```python
from build123d import *

# Parameters (mm, degrees)
SKETCH_1_R               = 12.5
EXTRUDE_1_DEPTH          = 6
SKETCH_4_R               = 1.15
CUT_EXTRUDE_2_DEPTH      = 19
SKETCH_3_R               = 7.5
CUT_EXTRUDE_3_DEPTH      = 5
CHAMFER_2_SIZE           = 0.7
SKETCH_8_R               = 17.454292773
SKETCH_8_R_2             = 8.65
CUT_EXTRUDE_4_DEPTH      = 3
PATTERN_CIRCULAR_2_COUNT = 6
SKETCH_2_R               = 7.34982993
EXTRUDE_2_DEPTH          = 10
SKETCH_9_R               = 1.85
CUT_EXTRUDE_5_DEPTH      = 0.3
CHAMFER_3_SIZE           = 0.7
PATTERN_CIRCULAR_3_COUNT = 6
CHAMFER_4_SIZE           = 0.7
SKETCH_10_W              = 4.08
SKETCH_10_H              = 4.08
CUT_EXTRUDE_6_DEPTH      = 8
FILLET_1_R               = 2
CHAMFER_5_SIZE           = 4.08


# Some blends are built 0.0001 mm under size
with BuildPart() as part:
    # 草图1 → 凸台-拉伸1 (new body)
    with BuildSketch(Plane(origin=(0, 0, 0), x_dir=(1, 0, 0), z_dir=(0, 1, 0))):
        with Locations(Location((0, 0, 0), (0, 0, 270))):
            Circle(SKETCH_1_R)
    extrude(amount=EXTRUDE_1_DEPTH)

    # 草图4 → 切除-拉伸2 (cut)
    with BuildSketch(Plane(origin=(0, 6, 0), x_dir=(1, 0, 0), z_dir=(0, 1, 0))):
        with Locations(Location((-10.5, 0, 0), (0, 0, 270))):
            Circle(SKETCH_4_R)
    cut_extrude_2 = extrude(amount=-CUT_EXTRUDE_2_DEPTH, mode=Mode.SUBTRACT)

    # 草图3 → 切除-拉伸3 (cut)
    with BuildSketch(Plane(origin=(0, 0, 0), x_dir=(-1, 0, 0), z_dir=(0, -1, 0))):
        with Locations(Location((0, 0, 0), (0, 0, 90))):
            Circle(SKETCH_3_R)
    extrude(amount=-CUT_EXTRUDE_3_DEPTH, mode=Mode.SUBTRACT)

    # 倒角2
    chamfer_2_edges = [part.edges().sort_by_distance(p)[0] for p in [
        (-10.5, 6, -1.15),
    ]]
    chamfer(chamfer_2_edges, length=CHAMFER_2_SIZE)

    # 草图8 → 切除-拉伸4 (cut)
    with BuildSketch(Plane(origin=(0, 6, 0), x_dir=(1, 0, 0), z_dir=(0, 1, 0))):
        Circle(SKETCH_8_R)
        with Locations(Location((0, 0, 0), (0, 0, 270))):
            Circle(SKETCH_8_R_2, mode=Mode.SUBTRACT)
    extrude(amount=-CUT_EXTRUDE_4_DEPTH, mode=Mode.SUBTRACT)

    # 阵列(圆周)2: 切除-拉伸2 ×6 about axis
    pattern_circular_2_axis = Axis((0, 0, 0), (0, 1, 0))
    for i in range(1, PATTERN_CIRCULAR_2_COUNT):
        add(cut_extrude_2.rotate(pattern_circular_2_axis, i * 360 / PATTERN_CIRCULAR_2_COUNT), mode=Mode.SUBTRACT)

    # 草图2 → 凸台-拉伸2 (add)
    with BuildSketch(Plane(origin=(0, 6, 0), x_dir=(1, 0, 0), z_dir=(0, 1, 0))):
        with Locations(Location((0, 0, 0), (0, 0, 270))):
            Circle(SKETCH_2_R)
    extrude(amount=EXTRUDE_2_DEPTH)

    # 草图9 → 切除-拉伸5 (cut)
    with BuildSketch(Plane(origin=(0, 3, 0), x_dir=(1, 0, 0), z_dir=(0, 1, 0))):
        with Locations(Location((-10.5, 0, 0), (0, 0, 270))):
            Circle(SKETCH_9_R)
    cut_extrude_5 = extrude(amount=-CUT_EXTRUDE_5_DEPTH, mode=Mode.SUBTRACT)

    # 倒角3
    chamfer_3_edges = [part.edges().sort_by_distance(p)[0] for p in [
        (-10.5, 2.7, -1.15),
    ]]
    chamfer(chamfer_3_edges, length=CHAMFER_3_SIZE - 0.0001)  # a hair under: the kernel refuses the full size

    # 阵列(圆周)3: 切除-拉伸5 ×6 about axis
    pattern_circular_3_axis = Axis((0, 0, 0), (0, 1, 0))
    for i in range(1, PATTERN_CIRCULAR_3_COUNT):
        add(cut_extrude_5.rotate(pattern_circular_3_axis, i * 360 / PATTERN_CIRCULAR_3_COUNT), mode=Mode.SUBTRACT)

    # 倒角4
    chamfer_4_edges = [part.edges().sort_by_distance(p)[0] for p in [
        (-4.254070786, 2.7, -9.66826674),
        (6.245929214, 2.7, -8.51826674),
        (10.5, 2.7, 1.15),
        (4.254070786, 2.7, 9.66826674),
        (-6.245929214, 2.7, 8.51826674),
    ]]
    chamfer(chamfer_4_edges, length=CHAMFER_4_SIZE - 0.0001)  # a hair under: the kernel refuses the full size

    # 草图10 → 切除-拉伸6 (cut)
    with BuildSketch(Plane(origin=(0, 16, 0), x_dir=(1, 0, 0), z_dir=(0, 1, 0))):
        Rectangle(SKETCH_10_W, SKETCH_10_H)
    extrude(amount=-CUT_EXTRUDE_6_DEPTH, mode=Mode.SUBTRACT)

    # 草图11 → 切除-旋转1 (revolve, cut)
    with BuildSketch(Plane(origin=(0, 0, 0), x_dir=(0, 0, -1), z_dir=(1, 0, 0)), mode=Mode.PRIVATE) as cut_revolve_1_sk:
        Polygon((-0.304897272, 10.075), (-10.874100718, 10.075), (-10.874100718, 6), (-3.64, 6), (-3.64, 7.875), (-2.04, 7.875), (-2.04, 9.125), (11.125701635, 9.125), (11.125701635, 10.075), align=None)
    revolve(cut_revolve_1_sk.sketch.rotate(Axis((0, 10.075, 0.304897272), (0, 0, 1)), 180), axis=Axis((0, 10.075, 0.304897272), (0, 0, 1)), mode=Mode.SUBTRACT)

    # 圆角1
    # the kernel refuses this fillet: 2 mm, written as the material it takes off along each edge
    with BuildSketch(Plane(origin=(0, 16, 0), x_dir=(0, 0, 1), z_dir=(-1, 0, 0))) as fillet_1_piece_1:
        with BuildLine():
            CenterArc((7.34982993 - FILLET_1_R, -FILLET_1_R), FILLET_1_R, 0, 90)
            Line((7.34982993 - FILLET_1_R, 0), (7.34982993, 0))
            Line((7.34982993, 0), (7.34982993, -FILLET_1_R))
        make_face()
    revolve(axis=Axis((0, 16, 0), (0, 1, 0)), mode=Mode.SUBTRACT)

    # 倒角5
    # the kernel refuses this chamfer: 4.08 mm, written as the material it adds along each edge
    with BuildSketch(Plane(origin=(2.04, 8, -2.04), x_dir=(0, 0.9996219169112968, -0.02749587661058642), z_dir=(-1, 0, 0))) as chamfer_5_piece_1_section:
        Polygon((CHAMFER_5_SIZE * 0.999621916911, -CHAMFER_5_SIZE * 0.0274958766106), (-CHAMFER_5_SIZE * 0.0274958766106, -CHAMFER_5_SIZE * 0.999621916911), (0, 0), align=None)
    chamfer_5_piece_1 = extrude(amount=4.08, mode=Mode.PRIVATE)
    chamfer_5_piece_1 = chamfer_5_piece_1 - Plane(origin=(0, 10.075, -1.478470711), x_dir=(0, 1, 0), z_dir=(0, 0, -1)) * Cylinder(0.95, 25, mode=Mode.PRIVATE)
    add(chamfer_5_piece_1)


solid = part.part
```
Geometry: final body of the model. Coordinates: model frame, mm. A direction names the side the tool comes from. Round coordinates to 2 decimals unless told otherwise and drop trailing zeros. Order: outer loops, then holes, each group sorted by start corner. A loop starts at its lowest first (then second) coordinate and runs counter-clockwise, first axis right, second up. Notation, with made-up numbers: (59.5, -19.75) -> (86.5, -19.75) arc R33 cw to (86.5, 11.25) -> close; hole circle Ø5 at (12, 30). An arc over 180 degrees is marked (long way). Use one line per item in the form item = value.
(1) Draft query along X for faces 4 (the face through (-7, 6, -3)), 5 (the face through (-0.661, 12.173, 2.829)). Return one class per face: pulls with the +X half, pulls with the -X half, needs draft (parallel to the pull), parting line crosses it, or undercut.
Results list:
face_4 = needs draft
face_5 = undercut
(2) Ray query, probe 1 along X at (y, z) = (1.5, 0); probe 2 along X at (y, z) = (4.5, 0); probe 3 along Z at (x, y) = (-4.5, 2.25). Return the intervals inside material, ascending. Write a range as [from, to].
Results list:
probe_1 = [-12.5, -11.65], [-9.35, -7.5], [7.5, 9.35], [11.65, 12.5]
probe_2 = [-8.65, -7.5], [7.5, 8.65]
probe_3 = [-11.66, -10.28], [-7.91, -6], [6, 7.91], [10.28, 11.66]
(3) Access query for faces 1 (the face through (0, 5, 0)), 2 (the face through (-6.81, 2.85, 8.1)), 3 (the face through (-11.623, 1.014, -0.249)). Directions: +Z, -Z, +X, -X, +Y, -Y. A direction counts if a zero-diameter tool reaches every point of the face in a straight line with its end or side. Return the directions, or none.
Results list:
face_1 = -Y
face_2 = +Y
face_3 = +Y, -Y
(4) First-contact query: pin 1 Ø5 at (x, y) = (1.5, 14) entering from -Z; pin 2 Ø2 at (y, z) = (1.5, -3) entering from -X; pin 3 Ø6 at (x, z) = (-5, -7) entering from +Y; pin 4 Ø1.4 at (x, z) = (5.25, -9.09) entering from -Y. Flat tips, straight axial feed; report the tip coordinate or a pass-through.
Results list:
pin_1 = -7.35
pin_2 = -12.34
pin_3 = 15.98
pin_4 = through
(5) Section B-B on x = -8. Return loops of the section in (y, z), and give its area (3 significant figures).
Results list:
outline = (0, -9.6) -> (3, -9.6) -> (3, -3.29) -> (6, -3.29) -> (6, 3.29) -> (3, 3.29) -> (3, 9.6) -> (0, 9.6) -> close
area = 77.4 mm^2
